Read the model definition and answer for the solid it produces. Units are mm, in the model's axes. Face numbers are marked on the shaded views. A direction names the side the tool comes from. Coordinates: 2 decimals unless noted, no trailing zeros. Order: outer loops, then holes, each group sorted by start corner. A loop starts at its lowest first (then second) coordinate and runs counter-clockwise, first axis right, second up. Notation, with made-up numbers: (3, 10) -> (46, 10) arc R8 ccw to (46, 14) -> close; hole circle Ø4 at (-18, 64.25). An arc over 180 degrees is marked (long way). Use CSV: the item, a comma, the result in double quotes.
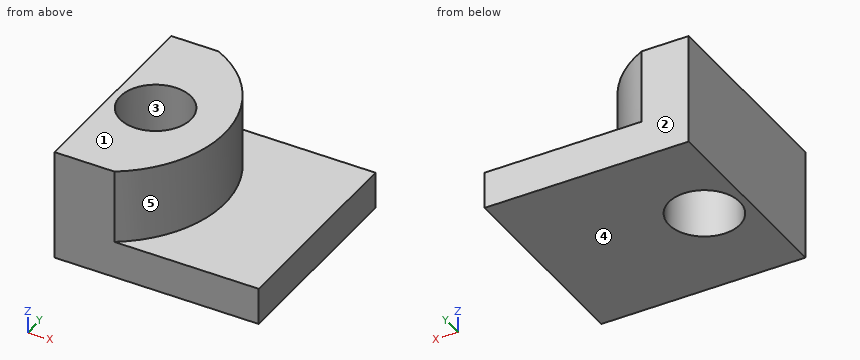
```python
from build123d import *

# Parameters (mm, degrees)
F0_W     = 69.85
F0_H     = 38.1
F1_DEPTH = 69.85
F3_DEPTH = 25.4
F4_R     = 12.130263
F5_DEPTH = 38.1


with BuildPart() as f1:
    # F0 (on Front) → F1 (new body)
    with BuildSketch(Plane.XZ):
        with Locations((34.925, 19.05)):
            Rectangle(F0_W, F0_H)
    extrude(amount=F1_DEPTH)

    # F2 (on face) → F3 (cut)
    with BuildSketch(Plane.XY.offset(38.1)):
        with BuildLine():
            ThreePointArc((16.126048, 0), (38.919005, -33.643201), (20.467674, -69.85))
            Line((20.467674, -69.85), (69.85, -69.85))
            Line((69.85, -69.85), (69.85, 0))
            Line((69.85, 0), (16.126048, 0))
        make_face()
    extrude(amount=-F3_DEPTH, mode=Mode.SUBTRACT)

    # F4 (on face) → F5 (cut)
    with BuildSketch(Plane.XY.offset(38.1)):
        with Locations((14.575467, -34.888081)):
            Circle(F4_R)
    extrude(amount=-F5_DEPTH, mode=Mode.SUBTRACT)


solid = f1.part
```
Item 1: Each of these flat-tipped pins is pushed along its axis until it touches: P1, Ø5, axis at y = -44, z = 21, coming from the +X side; P2, Ø19.5, axis at x = 14.58, y = -34.89, coming from the +Z side; P3, Ø4, axis at y = -19.5, z = 23.5, coming from the -X side; P4, Ø2, axis at y = -24.5, z = 23.5, coming from the +X side. Where does it stop, or does it pass through?
Return value:
P1,"stops at x = 38.63"
P2,"passes through"
P3,"stops at x = 0"
P4,"stops at x = 37.56"
Item 2: Find section C-C, the plane z = 26. Give the vertices of the cut face in (x, y).
Return value:
outline,"(0, -69.85) -> (20.47, -69.85) arc R39.96 ccw to (16.13, 0) -> (0, 0) -> close; hole circle Ø24.26 at (14.58, -34.89)"
Item 3: Find section D-D, the plane x = 30. Give the vertices of the cut face in (y, z), then the cut area to 3 significant figures.
Return value:
outline,"(-69.85, 0) -> (0, 0) -> (0, 12.7) -> (-10.86, 12.7) -> (-10.86, 38.1) -> (-61.38, 38.1) -> (-61.38, 12.7) -> (-69.85, 12.7) -> close"
area,"2,170 mm^2"
Item 4: Straight lines are drawn through the part: line 1 along Z through (x, y) = (36, -17); line 2 along X through (y, z) = (-32.5, 21); line 3 along Y through (x, z) = (20, 24). For each, find the intervals that lie inside material, in ascending order.
Return value:
line 1,"z = 0 to 12.7"
line 2,"x = 0 to 2.68, 26.47 to 38.83"
line 3,"y = -69.85 to -45.74, -24.04 to -2.1"
Item 5: The mould has two halves that part along Y. Classify the marked faces 1, 2 and 3: +Y half, -Y half, draft (parallel to the pull), parting line (faces both ways), or undercut.
Return value:
face 1,"draft"
face 2,"+Y half"
face 3,"undercut"
Item 6: Find section A-A, the plane x = 23. Give the vertices of the cut face in (y, z).
Return value:
outline,"(-69.85, 0) -> (-43.62, 0) -> (-43.62, 38.1) -> (-68.1, 38.1) -> (-68.1, 12.7) -> (-69.85, 12.7) -> close; (-26.16, 0) -> (0, 0) -> (0, 12.7) -> (-4.14, 12.7) -> (-4.14, 38.1) -> (-26.16, 38.1) -> close"
Item 7: Find section B-B, the plane y = -33. Give the vertices of the cut face in (x, z), then the cut area to 3 significant figures.
Return value:
outline,"(0, 0) -> (2.59, 0) -> (2.59, 38.1) -> (0, 38.1) -> close; (26.56, 0) -> (69.85, 0) -> (69.85, 12.7) -> (38.87, 12.7) -> (38.87, 38.1) -> (26.56, 38.1) -> close"
area,"961 mm^2"
Item 8: A tool of negligible diameter and unlimited length cuts with its end or side. For the marked faces 4 and 5, from which of +Z, -Z, +X, -X, +Y, -Y can it reach the whole face along a straight path? Write none if from no direction.
Return value:
face 4,"-Z, +X, -X, +Y, -Y"
face 5,"+Z, +X"
